from build123d import *

# Parameters (mm, degrees)
SKETCH1_W           = 39
SKETCH1_H           = 21
BOSS_EXTRUDE1_DEPTH = 11.5
SKETCH3_W           = 37
SKETCH3_H           = 19
CUT_EXTRUDE2_DEPTH  = 4
FILLET1_R           = 1
FILLET2_R           = 1
SKETCH5_R           = 4.5
BOSS_EXTRUDE2_DEPTH = 2
SKETCH6_R           = 3.5
CUT_EXTRUDE4_DEPTH  = 9.5
SKETCH7_R           = 4.5
BOSS_EXTRUDE3_DEPTH = 1
SKETCH8_R           = 1.75
CUT_EXTRUDE5_DEPTH  = 1
CUT_EXTRUDE6_DEPTH  = 1
CUT_EXTRUDE7_DEPTH  = 39


with BuildPart() as part:
    # Sketch1 → Boss-Extrude1 (new body)
    with BuildSketch(Plane(origin=(0, 0, 0), x_dir=(1, 0, 0), z_dir=(0, 1, 0))):
        with Locations((19.5, 10.5)):
            Rectangle(SKETCH1_W, SKETCH1_H)
    extrude(amount=BOSS_EXTRUDE1_DEPTH)

    # Sketch3 → Cut-Extrude2 (cut)
    with BuildSketch(Plane(origin=(0, 11.5, 0), x_dir=(1, 0, 0), z_dir=(0, 1, 0))):
        with Locations((19.5, 10.5)):
            Rectangle(SKETCH3_W, SKETCH3_H)
    extrude(amount=-CUT_EXTRUDE2_DEPTH, mode=Mode.SUBTRACT)

    # Fillet1
    fillet1_edges = [part.edges().sort_by_distance(p)[0] for p in [
        (0, 5.75, -21),
        (39, 5.75, -21),
        (39, 5.75, 0),
        (0, 5.75, 0),
    ]]
    fillet(fillet1_edges, radius=FILLET1_R)

    # Fillet2
    fillet2_edges = [part.edges().sort_by_distance(p)[0] for p in [
        (19.5, 0, 0),
        (0, 0, -10.5),
        (19.5, 0, -21),
        (39, 0, -10.5),
        (0.292893219, 0, -20.707106781),
        (38.707106781, 0, -20.707106781),
        (38.707106781, 0, -0.292893219),
        (0.292893219, 0, -0.292893219),
    ]]
    fillet(fillet2_edges, radius=FILLET2_R)

    # Sketch5 → Boss-Extrude2 (add)
    with BuildSketch(Plane(origin=(0, 7.5, 0), x_dir=(1, 0, 0), z_dir=(0, 1, 0))):
        with Locations((28.01, 10.44)):
            Circle(SKETCH5_R)
    extrude(amount=BOSS_EXTRUDE2_DEPTH)

    # Sketch6 → Cut-Extrude4 (cut)
    with BuildSketch(Plane(origin=(0, 9.5, 0), x_dir=(1, 0, 0), z_dir=(0, 1, 0))):
        with Locations((28.01, 10.44)):
            Circle(SKETCH6_R)
    extrude(amount=-CUT_EXTRUDE4_DEPTH, mode=Mode.SUBTRACT)

    # Sketch7 → Boss-Extrude3 (add)
    with BuildSketch(Plane(origin=(0, 9.5, 0), x_dir=(1, 0, 0), z_dir=(0, 1, 0))):
        with Locations((28.01, 10.44)):
            Circle(SKETCH7_R)
    extrude(amount=-BOSS_EXTRUDE3_DEPTH)

    # Sketch8 → Cut-Extrude5 (cut)
    with BuildSketch(Plane(origin=(0, 9.5, 0), x_dir=(1, 0, 0), z_dir=(0, 1, 0))):
        with Locations((28.01, 10.44)):
            Circle(SKETCH8_R)
    extrude(amount=-CUT_EXTRUDE5_DEPTH, mode=Mode.SUBTRACT)

    # Sketch9 → Cut-Extrude6 (cut)
    with BuildSketch(Plane(origin=(39, 0, 0), x_dir=(0, 0, -1), z_dir=(1, 0, 0))):
        with BuildLine():
            Line((8.5, 11.5), (12.5, 11.5))
            ThreePointArc((12.5, 11.5), (10.5, 9.5), (8.5, 11.5))
        make_face()
    extrude(amount=-CUT_EXTRUDE6_DEPTH, mode=Mode.SUBTRACT)

    # Sketch4 → Cut-Extrude7 (cut)
    with BuildSketch(Plane.ZY):
        with BuildLine():
            Line((-14.208099244, 0), (-6.791900756, 0))
            ThreePointArc((-6.791900756, 0), (-10.5, 5.5), (-14.208099244, 0))
        make_face()
    extrude(amount=-CUT_EXTRUDE7_DEPTH, mode=Mode.SUBTRACT)


solid = part.part
Model file for the job. Use its own axes, mm. A direction names the side the tool comes from. Give positions to 0.01 mm unless a question says otherwise; leave off trailing zeros. Order: outer loops, then holes, each group sorted by start corner. A loop starts at its lowest first (then second) coordinate and runs counter-clockwise, first axis right, second up. Notation, with made-up numbers: (23.5, -30.5) -> (34.5, -30.5) arc R27 ccw to (34.5, 3.5) -> close; hole circle Ø7 at (-7, 80). An arc over 180 degrees is marked (long way). Use CSV: the item, a comma, the result in double quotes.
1. Band-saw the part on B-B, the plane y = 7. Give the cut face in (x, z).
Outcome:
outline,"(0, -20) arc R1 ccw to (1, -21) -> (38, -21) arc R1 ccw to (39, -20) -> (39, -1) arc R1 ccw to (38, 0) -> (1, 0) arc R1 ccw to (0, -1) -> close; hole circle Ø7 at (28.01, -10.44)"
2. Drill centre lines: line 1 along X through (y, z) = (9.3, -10.44); line 2 along Z through (x, y) = (28.01, 9.2); line 3 along Z through (x, y) = (29.5, 10.75). Where is each one in solid material? Low to high. Write a range as from..to.
Outcome:
line 1,"0..1, 23.51..26.26, 29.76..32.51, 38..39"
line 2,"-21..-20, -14.94..-12.19, -8.69..-5.94, -1..0"
line 3,"-21..-20, -1..0"
3. Band-saw the part on A-A, the plane y = 1.5. Give the cut face in (x, z), then the cut area to 3 significant figures.
Outcome:
outline,"(0, -20) arc R1 ccw to (1, -21) -> (38, -21) arc R1 ccw to (39, -20) -> (39, -14.5) -> (0, -14.5) -> close; (0, -6.5) -> (39, -6.5) -> (39, -1) arc R1 ccw to (38, 0) -> (1, 0) arc R1 ccw to (0, -1) -> close"
area,"506 mm²"
4. Mould opens along Z. For faces 5 (the cylindrical face through (38.699, 6.324, -20.715)), 6 (the cylindrical face through (0.301, 0.285, -3.855)), 7 (the flat face through (19, 7.5, -11)) say: +Z half, -Z half, draft (parallel to the pull), parting line (faces both ways), or undercut.
Outcome:
face 5,"-Z half"
face 6,"draft"
face 7,"undercut"
5. Band-saw the part on C-C, the plane x = 28.01. Give the cut face in (y, z), then the cut area to 3 significant figures.
Outcome:
outline,"(0, -20) arc R1 ccw to (1, -21) -> (11.5, -21) -> (11.5, -20) -> (7.5, -20) -> (7.5, -14.94) -> (9.5, -14.94) -> (9.5, -12.19) -> (8.5, -12.19) -> (8.5, -13.94) -> (3.54, -13.94) arc R4 cw to (0, -14.21) -> close; (0, -6.79) arc R4 cw to (3.32, -6.94) -> (8.5, -6.94) -> (8.5, -8.69) -> (9.5, -8.69) -> (9.5, -5.94) -> (7.5, -5.94) -> (7.5, -1) -> (11.5, -1) -> (11.5, 0) -> (1, 0) arc R1 ccw to (0, -1) -> close"
area,"118 mm²"
6. Drop flat-ended pins along their axis: pin 1 (8 mm diameter, centred on x = 10.5, z = -9, fed in from -Y); pin 2 (5.5 mm diameter, centred on x = 28.01, z = -10.44, fed in from +Y); pin 3 (1 mm diameter, centred on x = 10, z = -11, fed in from -Y); pin 4 (4 mm diameter, centred on x = 22, z = -11.5, fed in from -Y). Give the stop position or say it passes through.
Outcome:
pin 1,"y = 0"
pin 2,"y = 9.5"
pin 3,"y = 5.37"
pin 4,"y = 4.15"
7. 3-axis set-ups, long thin cutter, end or side, ignore diameter. For faces 1 (the cylindrical face through (23.514, 8.486, -10.638)), 2 (the cylindrical face through (38.699, 0.285, -17.145)), 3 (the flat face through (26, 8.5, -10)), 4 (the cylindrical face through (38.5, 9.5, -10.5)): which of +Z, -Z, +X, -X, +Y, -Y reach the whole face in a straight line?
Outcome:
face 1,"+Y"
face 2,"+Z, -Z, +X, -Y"
face 3,"-Y"
face 4,"+X, +Y"
8. Band-saw the part on D-D, the plane z = -10. Give the cut face in (x, y), then the cut area to 3 significant figures.
Outcome:
outline,"(0, 5.47) -> (24.54, 5.47) -> (24.54, 8.5) -> (26.32, 8.5) -> (26.32, 9.5) -> (23.53, 9.5) -> (23.53, 7.5) -> (1, 7.5) -> (1, 11.5) -> (0, 11.5) -> close; (29.7, 8.5) -> (31.48, 8.5) -> (31.48, 5.47) -> (39, 5.47) -> (39, 9.56) -> (38, 9.56) -> (38, 7.5) -> (32.49, 7.5) -> (32.49, 9.5) -> (29.7, 9.5) -> close"
area,"78.8 mm²"
